from build123d import *


with BuildPart() as f1:
    # F0 (on Front) → F1 (revolve)
    with BuildSketch(Plane.XZ):
        with BuildLine():
            Line((46.6274327665, 20.4293505417), (52.3332152067, 25.8130880211))
            add(Edge.make_bspline(
                [(52.3332152067, 25.8130880211), (52.6873531533, 26.0396653478), (53.287973728, 26.3773534836), (53.9061448765, 26.4795545854), (54.1609440093, 26.4919212472)],
                knots=[0.0753740232, 0.0753740232, 0.0753740232, 0.0753740232, 0.236653892, 0.3473965491, 0.3473965491, 0.3473965491, 0.3473965491], degree=3))
            Line((54.1609440093, 26.4919212472), (54.1609440093, 28.4919212472))
            Line((54.1609440093, 28.4919212472), (0, 28.4919212472))
            Line((0, 28.4919212472), (-2, 28.4919212472))
            Line((-2, 28.4919212472), (-2, 0))
            Line((-2, 0), (0, 0))
            Line((0, 0), (0, 12.5))
            Line((0, 12.5), (26, 12.5))
            ThreePointArc((26, 12.5), (26.7071067812, 12.7928932188), (27, 13.5))
            Line((27, 13.5), (27, 15))
            ThreePointArc((27, 15), (27.2928932188, 15.7071067812), (28, 16))
            Line((28, 16), (44.9999994072, 16))
            ThreePointArc((44.9999994072, 16), (45.707106398, 16.2928934284), (45.9999994072, 17.0000005928))
            Line((45.9999994072, 17.0000005928), (45.9999982367, 18.9746813235))
            ThreePointArc((45.9999982367, 18.9746813235), (46.1635437461, 19.7667886958), (46.6274327665, 20.4293505417))
        make_face()
    revolve(axis=Axis((19.5, 0, 0), (-1, 0, 0)))


solid = f1.part
Model file for the job. Use its own axes, mm. A direction names the side the tool comes from. Coordinates: 2 decimals unless noted, no trailing zeros. Order: outer loops, then holes, each group sorted by start corner. A loop starts at its lowest first (then second) coordinate and runs counter-clockwise, first axis right, second up. Notation, with made-up numbers: M 33,29 L 72,29 A10 ccw 72,42 Z; hole C 78,-30 d2. An arc over 180 degrees is marked long. Return JSON: item names as keys, results as strings.
1. Saw through at B-B (x = 48). Give the cut face in (y, z).
Ans:
{"outline": "C 0,0 d56.98; hole C 0,0 d43.45"}
2. Saw through at A-A (x = 14). Give the cut face in (y, z).
Ans:
{"outline": "C 0,0 d56.98; hole C 0,0 d25"}
3. Tool access for faces 1 (the face through (54.161, -19, -19)), 2 (the face through (0, 0, 0)): list every direction of +Z, -Z, +X, -X, +Y, -Y with a clear straight run to the whole face (end or side of a thin tool).
Ans:
{"face 1": "+Z, -Z, +X, +Y, -Y", "face 2": "+X"}
4. Flat gauge pins, fed straight in: pin 1 (10 mm diameter, centred on x = 42.5, y = -9.5, fed in from +Z); pin 2 (1 mm diameter, centred on x = 29, y = 15.5, fed in from +Z); pin 3 (1.5 mm diameter, centred on x = 42, z = -20.5, fed in from -Y). Where does each tip first touch, or does it go through?
Ans:
{"pin 1": "z = 28.13", "pin 2": "z = 24.22", "pin 3": "y = -20.54"}
5. Pull direction Z, two halves, no side cores. Call faces 3 (the face through (25.687, 1.253, -28.464)), 4 (the face through (36.62, -15.62, -3.47)), 5 (the face through (46.984, 0.913, -20.746)), 6 (the face through (-2, 0, 0)): +Z half, -Z half, draft (parallel to the pull), parting line (faces both ways), or undercut.
Ans:
{"face 3": "parting line", "face 4": "undercut", "face 5": "undercut", "face 6": "draft"}
6. Drill centre lines: probe 1 along Y at (x, z) = (9, 0); probe 2 along Y at (x, z) = (38, 0); probe 3 along Z at (x, y) = (20, 5). Where is each one in solid material? Low to high.
Ans:
{"probe 1": "-28.49 to -12.5, 12.5 to 28.49", "probe 2": "-28.49 to -16, 16 to 28.49", "probe 3": "-28.05 to -11.46, 11.46 to 28.05"}
